Study the drawing (mm; zero at the part's minimum x, y, z) and answer. Round coordinates to 2 decimals unless told otherwise and drop trailing zeros. Loops run counter-clockwise (first coordinate to the right, second up) from the corner with the lowest first, then second, coordinate; pieces in that order, holes last. Notation, with made-up numbers: M 54,23 L 61,23 A21 ccw 61,32 Z; hole C 60.5,-32.5 d3. An arc over 180 degrees is marked long. Put each result on its own line as item: value. Start each with the question number.
(1) Section C-C, the plane z = 65.5 is taken. Determine the outline of the cut face in (x, y).
(2) Straight lines are drawn through the part: line 1 (Z direction, x = 54, y = 1.25) (1 decimal); line 2 (Z direction, x = 18, y = 1.5) (1 decimal); line 3 (Z direction, x = 122.5, y = 1.05) (1 decimal). For each, find the intervals that lie inside material, in ascending order.
(3) Flat-ended cylindrical pins translate along their axes: P1, Ø4.5, axis at x = 45.03, z = 108.74, coming from the +Y side; P2, Ø1.2, axis at y = 1.5, z = 58.5, coming from the -X side. Find the tip coordinate at first contact, or state that the pin passes through.
(4) Section B-B, the plane y = 2 is taken. Count the separate pieces of the cut face and the enclosed holes in it, then the cut area to 3 significant figures.
(5) Section A-A, the plane x = 80 is taken. Determine the outline of the cut face in (y, z) (1 decimal).
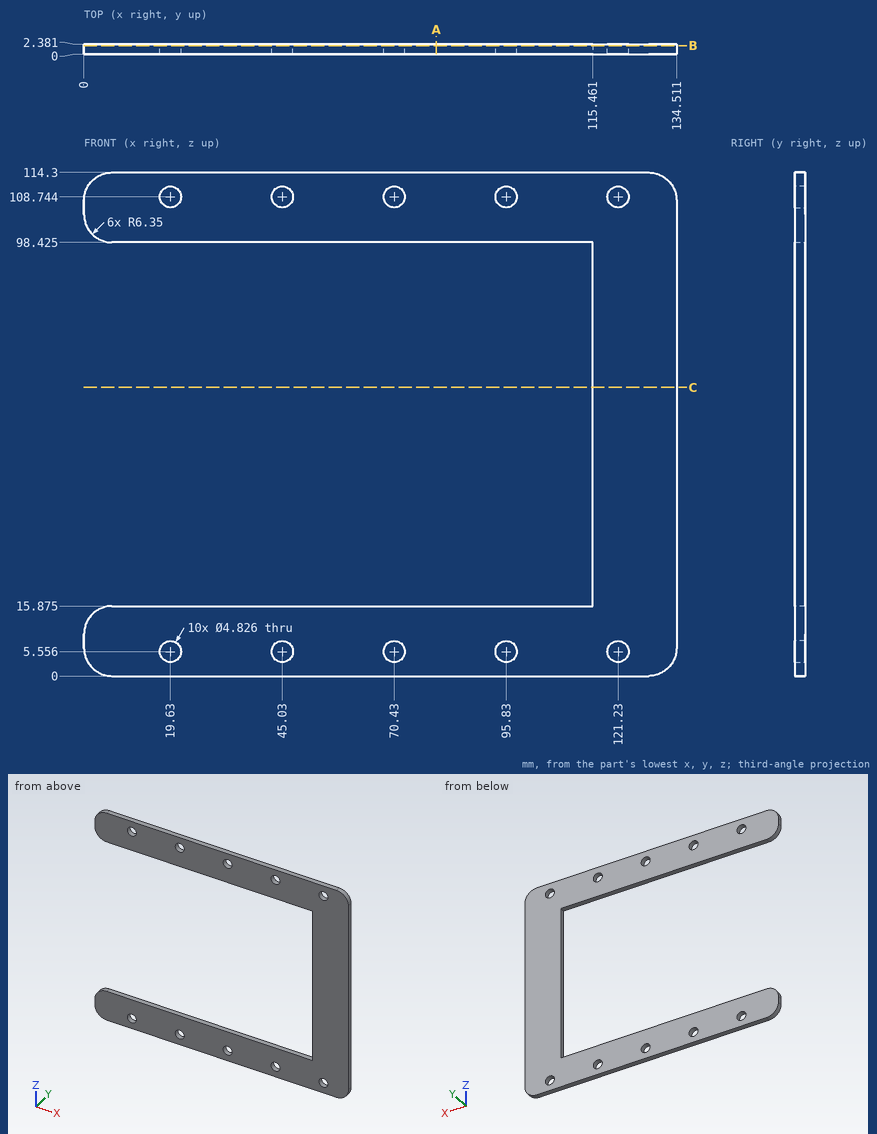
Recorded:
1. outline: M 115.46,0 L 134.51,0 L 134.51,2.38 L 115.46,2.38 Z
2. line 1: z = 0 to 15.9, 98.4 to 114.3
2. line 2: z = 0 to 3.8, 7.3 to 15.9, 98.4 to 107, 110.5 to 114.3
2. line 3: z = 0 to 3.5, 7.6 to 106.7, 110.8 to 114.3
3. P1: passes through
3. P2: stops at x = 115.46
4. separate pieces: 1
4. enclosed holes: 10
4. area: 5,610 mm²
5. outline: M 0,0 L 2.4,0 L 2.4,15.9 L 0,15.9 Z; M 0,98.4 L 2.4,98.4 L 2.4,114.3 L 0,114.3 Z
